Geometry: see drawing. Coordinates: mm, zero at the bounding-box minimum. A direction names the side the tool comes from. Give positions to 0.01 mm unless a question says otherwise; leave off trailing zeros. Write each loop counter-clockwise with the first axis right and the second up, starting at its lowest first coordinate (ties: lowest second). Pieces come first, ordered by that corner, then holes. Notation, with made-up numbers: (41, -21) - (45, -21) arc R16 cw to (45, 4) - close; hole circle Ø6 at (39.25, 62.5). An arc over 180 degrees is marked (long way). Return JSON: item names as keys, results as strings.
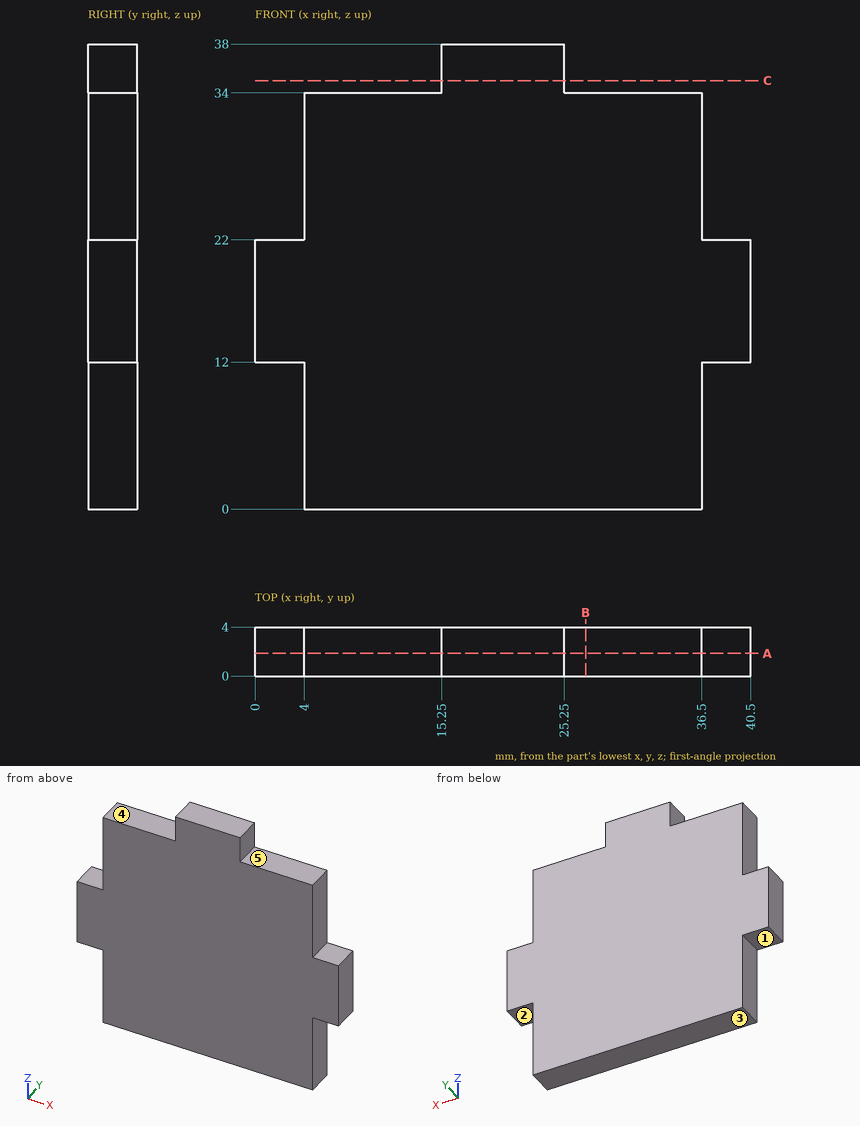
Q1. Section query A-A, the plane y = 1.85. Return the cut outline in (x, z).
Answer key:
{"outline": "(0, 12) - (4, 12) - (4, 0) - (36.5, 0) - (36.5, 12) - (40.5, 12) - (40.5, 22) - (36.5, 22) - (36.5, 34) - (25.25, 34) - (25.25, 38) - (15.25, 38) - (15.25, 34) - (4, 34) - (4, 22) - (0, 22) - close"}
Q2. Section query B-B, the plane x = 27. Return the cut outline in (y, z), plus the area to 3 significant figures.
Answer key:
{"outline": "(0, 0) - (4, 0) - (4, 34) - (0, 34) - close", "area": "136 mm^2"}
Q3. Section query C-C, the plane z = 35. Return the cut outline in (x, y).
Answer key:
{"outline": "(15.25, 0) - (25.25, 0) - (25.25, 4) - (15.25, 4) - close"}
Q4. Pin query (flat end, axial travel): P1, Ø2, axis at x = 38.5, y = 3, coming from the -Z side; P2, Ø1, axis at y = 2, z = 31.5, coming from the -X side; P3, Ø2, axis at x = 7, y = 1.5, coming from the +Z side. Return the tip coordinate at first contact, or that it passes through.
Answer key:
{"P1": "stops at z = 12", "P2": "stops at x = 4", "P3": "stops at z = 34"}
Q5. Set-up query: the marked faces 1, 2, 3, 4 and 5. Return all of +Z, -Z, +X, -X, +Y, -Y with unobstructed straight access to the full face (end or side cutting, diameter ignored); none if empty.
Answer key:
{"face 1": "-Z, -X, +Y, -Y", "face 2": "-Z, +X, +Y, -Y", "face 3": "-Z, +X, -X, +Y, -Y", "face 4": "+Z, -X, +Y, -Y", "face 5": "+Z, +X, +Y, -Y"}
Q6. Material intervals for probe 1 along X at (y, z) = (1.3, 23.5); probe 2 along Z at (x, y) = (31, 1.2); probe 3 along X at (y, z) = (0.75, 36), sorted ascending. Write a range as [from, to].
Answer key:
{"probe 1": "x = [4, 36.5]", "probe 2": "z = [0, 34]", "probe 3": "x = [15.25, 25.25]"}
